For this review, take the finished solid that the model builds, in its own axes (mm). A direction names the side the tool comes from. Round coordinates to 2 decimals unless told otherwise and drop trailing zeros. Order: outer loops, then holes, each group sorted by start corner. A loop starts at its lowest first (then second) coordinate and runs counter-clockwise, first axis right, second up.
```python
from build123d import *

# Parameters (mm, degrees)
SKETCH1_W                                  = 70
SKETCH1_H                                  = 36
BOSS_EXTRUDE1_DEPTH                        = 8
SKETCH2_W                                  = 5.5
SKETCH2_H                                  = 8
CUT_EXTRUDE1_DEPTH                         = 41.162171256
CBORE_START                                = 33
CBORE_FOR_M3_CHEESE_HEAD_SCREW1_OUTLINE_R  = 3.25
CBORE_FOR_M3_CHEESE_HEAD_SCREW1_DEPTH      = 2
CBORE_START_2                              = 30.25
CBORE_FOR_M3_CHEESE_HEAD_SCREW1_2_OUTLIN_R = 1.7
CBORE_FOR_M3_CHEESE_HEAD_SCREW1_2_DEPTH    = 2.75
CUT_EXTRUDE2_DEPTH                         = 3
MIRROR2_START                              = 33
MIRROR2_COPY_1_SKETCH_R                    = 3.25
MIRROR2_COPY_1_DEPTH                       = 2
MIRROR2_START_2                            = 30.25
MIRROR2_COPY_2_SKETCH_R                    = 1.7
MIRROR2_COPY_2_DEPTH                       = 2.75
MIRROR2_COPY_3_DEPTH                       = 3
MIRROR2_COPY_4_SKETCH_R                    = 1.7
MIRROR2_COPY_4_DEPTH                       = 2.75
CHAMFER1_SIZE                              = 2


# Read off the part's stored shape, not the designer's step: CBORE for M3 Cheese Head Screw1
with BuildPart() as part:
    # Sketch1 → Boss-Extrude1 (new body)
    with BuildSketch(Plane(origin=(0, 0, 0), x_dir=(1, 0, 0), z_dir=(0, 1, 0))):
        Rectangle(SKETCH1_W, SKETCH1_H)
    extrude(amount=BOSS_EXTRUDE1_DEPTH)

    # Sketch2 → Cut-Extrude1 (cut, through all)
    with BuildSketch(Plane(origin=(0, 8, 0), x_dir=(1, 0, 0), z_dir=(0, 1, 0))):
        with Locations((-27.5, 14)):
            Rectangle(SKETCH2_W, SKETCH2_H)
        with Locations((27.5, 14)):
            Rectangle(SKETCH2_W, SKETCH2_H)
    cut_extrude1 = extrude(amount=-CUT_EXTRUDE1_DEPTH, mode=Mode.SUBTRACT)

    # CBORE for M3 Cheese Head Screw1 outline → CBORE for M3 Cheese Head Screw1 (cut)
    with BuildSketch(Plane.YZ.offset(CBORE_START)):
        with Locations((4, -14)):
            Circle(CBORE_FOR_M3_CHEESE_HEAD_SCREW1_OUTLINE_R)
    cbore_for_m3_cheese_head_screw1 = extrude(amount=CBORE_FOR_M3_CHEESE_HEAD_SCREW1_DEPTH, mode=Mode.SUBTRACT)

    # CBORE for M3 Cheese Head Screw1 2 outlin → CBORE for M3 Cheese Head Screw1 2 (cut)
    with BuildSketch(Plane.YZ.offset(CBORE_START_2)):
        with Locations((4, -14)):
            Circle(CBORE_FOR_M3_CHEESE_HEAD_SCREW1_2_OUTLIN_R)
    cbore_for_m3_cheese_head_screw1_2 = extrude(amount=CBORE_FOR_M3_CHEESE_HEAD_SCREW1_2_DEPTH, mode=Mode.SUBTRACT)

    # Sketch9 → Cut-Extrude2 (cut)
    with BuildSketch(Plane(origin=(24.75, 0, 0), x_dir=(0, 0, -1), z_dir=(1, 0, 0))):
        Polygon((15.616580754, 6.8), (12.383419246, 6.8), (10.766838493, 4), (12.383419246, 1.2), (15.616580754, 1.2), (17.233161507, 4), align=None)
    cut_extrude2 = extrude(amount=-CUT_EXTRUDE2_DEPTH, mode=Mode.SUBTRACT)

    # Mirror1: CBORE for M3 Cheese Head Screw1, CBORE for M3 Cheese Head Screw1 2, Cut-Extrude2 across plane
    add(cbore_for_m3_cheese_head_screw1.mirror(Plane(origin=(0, 0, 0), x_dir=(0, 0, 1), z_dir=(1, 0, 0))), mode=Mode.SUBTRACT)
    add(cbore_for_m3_cheese_head_screw1_2.mirror(Plane(origin=(0, 0, 0), x_dir=(0, 0, 1), z_dir=(1, 0, 0))), mode=Mode.SUBTRACT)
    add(cut_extrude2.mirror(Plane(origin=(0, 0, 0), x_dir=(0, 0, 1), z_dir=(1, 0, 0))), mode=Mode.SUBTRACT)

    # Mirror2: Cut-Extrude1, CBORE for M3 Cheese Head Screw1, CBORE for M3 Cheese Head Screw1 2, Cut-Extrude2 across plane
    add(cut_extrude1.mirror(Plane.XY), mode=Mode.SUBTRACT)
    add(cbore_for_m3_cheese_head_screw1.mirror(Plane.XY), mode=Mode.SUBTRACT)
    add(cbore_for_m3_cheese_head_screw1_2.mirror(Plane.XY), mode=Mode.SUBTRACT)
    add(cut_extrude2.mirror(Plane.XY), mode=Mode.SUBTRACT)

    # Mirror2 copy 1 sketch → Mirror2 copy 1 (cut)
    with BuildSketch(Plane(origin=(0, 0, 0), x_dir=(0, 1, 0), z_dir=(-1, 0, 0)).offset(MIRROR2_START)):
        with Locations((4, -14)):
            Circle(MIRROR2_COPY_1_SKETCH_R)
    extrude(amount=MIRROR2_COPY_1_DEPTH, mode=Mode.SUBTRACT)

    # Mirror2 copy 2 sketch → Mirror2 copy 2 (cut)
    with BuildSketch(Plane(origin=(0, 0, 0), x_dir=(0, 1, 0), z_dir=(-1, 0, 0)).offset(MIRROR2_START_2)):
        with Locations((4, -14)):
            Circle(MIRROR2_COPY_2_SKETCH_R)
    extrude(amount=MIRROR2_COPY_2_DEPTH, mode=Mode.SUBTRACT)

    # Mirror2 copy 3 sketch → Mirror2 copy 3 (cut)
    with BuildSketch(Plane.ZY.offset(24.75)):
        Polygon((15.616580754, 6.8), (12.383419246, 6.8), (10.766838493, 4), (12.383419246, 1.2), (15.616580754, 1.2), (17.233161507, 4), align=None)
    extrude(amount=-MIRROR2_COPY_3_DEPTH, mode=Mode.SUBTRACT)

    # Mirror2 copy 4 sketch → Mirror2 copy 4 (cut)
    with BuildSketch(Plane.YZ.offset(MIRROR2_START_2)):
        with Locations((4, 14)):
            Circle(MIRROR2_COPY_4_SKETCH_R)
    extrude(amount=MIRROR2_COPY_4_DEPTH, mode=Mode.SUBTRACT)

    # Chamfer1
    chamfer1_edges = [part.edges().sort_by_distance(p)[0] for p in [
        (32.625, 0, 18),
        (32.625, 8, 18),
        (-32.625, 8, 18),
        (-32.625, 0, -18),
        (-32.625, 8, -18),
        (0, 0, -18),
        (0, 8, -18),
        (-32.625, 0, 18),
        (32.625, 0, -18),
        (32.625, 8, -18),
        (0, 0, 18),
        (0, 8, 18),
    ]]
    chamfer(chamfer1_edges, length=CHAMFER1_SIZE)


solid = part.part
```
Q1. Take a section at A-A, the plane x = 17.5. State the section outline as (y, z) points, plus the area to 3 significant figures.
Q2. Tool access review of faces 1 (the face through (-31.61, 5.62, 13.49)), 2 (the face through (30.25, 4, -12)), 3 (the face through (-23, 6.8, 14)): name each direction out of +Z, -Z, +X, -X, +Y, -Y from which nothing blocks a thin tool from reaching the whole face with its end or side.
Q3. Take a section at C-C, the plane x = -29. State the section outline as (y, z) points, plus the area to 3 significant figures.
Q4. Take a section at B-B, the plane y = 3. Count the separate pieces of the cut face and the enclosed holes in it, plus the area to 3 significant figures.
Q5. Mouldability with a two-part tool opening along Y and no side actions: class faces 4 (the face through (33, 1, 17)), 5 (the face through (33, 7, 17)), 6 (the face through (33, 4, -18)), 7 (the face through (-23.271, 5.42, 11.586)) as +Y half, -Y half, draft (parallel to the pull), parting line (faces both ways), or undercut.
Q6. Wall thickness on line 1 (Z direction, x = 30.8, y = 4); line 2 (Z direction, x = 34.05, y = 4); line 3 (Y direction, x = -33.85, z = 14): over which ranges is each line inside the solid? List them lowest first.
Q7. Clearance check with flat-ended pins moving along their axes: pin 1 (3 mm diameter, centred on x = 26.5, y = 4.5, fed in from -Z); pin 2 (2.5 mm diameter, centred on y = 4.5, z = 12.5, fed in from -X); pin 3 (4 mm diameter, centred on y = 3.5, z = 13.5, fed in from +X). State where each tip first meets the part, or that it passes through.
Working result:
1. outline: (0, -16) - (2, -18) - (6, -18) - (8, -16) - (8, 16) - (6, 18) - (2, 18) - (0, 16) - close
1. area: 280 mm2
2. face 1: -X
2. face 2: -Z, +Y, -Y
2. face 3: none
3. outline: (0, -10) - (8, -10) - (8, 10) - (0, 10) - close
3. area: 160 mm2
4. separate pieces: 5
4. enclosed holes: 0
4. area: 2,200 mm2
5. face 4: -Y half
5. face 5: +Y half
5. face 6: draft
5. face 7: undercut
6. line 1: z = -18 to -15.7, -12.3 to 12.3, 15.7 to 18
6. line 2: z = -18 to -17.25, -10.75 to 10.75, 17.25 to 18
6. line 3: y = 0 to 0.75, 7.25 to 8
7. pin 1: stops at z = -10
7. pin 2: stops at x = -33
7. pin 3: stops at x = 33
